Geometry: final body of the model. Coordinates: model frame, mm. A direction names the side the tool comes from. Give positions to 0.01 mm unless a question says otherwise; leave off trailing zeros. Write each loop counter-clockwise with the first axis right and the second up, starting at its lowest first coordinate (ties: lowest second). Pieces come first, ordered by that corner, then holes. Notation, with made-up numbers: M 79.25,76 L 124.25,76 A32 cw 124.25,105 Z; hole C -12.5,54 d4. An arc over 180 degrees is marked long. One line per question, with ' | ' between items.
from build123d import *

# Parameters (mm, degrees)
SKIZZE1_W                            = 238.8
SKIZZE1_H                            = 154.7
AUFSATZ_LINEAR_AUSTRAGEN1_DEPTH      = 3
SKIZZE2_W                            = 238.8
SKIZZE2_H                            = 154.7
SKIZZE2_W_2                          = 204.8
SKIZZE2_H_2                          = 120.7
SCHNITT_LINEAR_AUSTRAGEN2_DEPTH      = 2
VERRUNDUNG3_R                        = 8
F_3_0_3_DURCHMESSER_BOHRUNG1_D       = 3
SKIZZE6_W                            = 52
SKIZZE6_H                            = 44.7
SCHNITT_LINEAR_AUSTRAGEN3_DEPTH      = 285.546182543
SKIZZE7_W                            = 131.8
SKIZZE7_H                            = 87.7
SCHNITT_LINEAR_AUSTRAGEN4_DEPTH      = 285.546182543
SKIZZE5_W                            = 137.8
SKIZZE5_H                            = 93.7
SKIZZE5_W_2                          = 131.8
SKIZZE5_H_2                          = 87.7
AUFSATZ_LINEAR_AUSTRAGEN2_DEPTH      = 25
SCHNITT_LINEAR_AUSTRAGEN5_REACH      = 246.152
SKIZZE8_W                            = 40.7
SKIZZE8_H                            = 2
SKIZZE9_W                            = 43
SKIZZE9_H                            = 23
AUFSATZ_LINEAR_AUSTRAGEN3_DEPTH      = 4
F_3_4_3_4_DURCHMESSER_BOHRUNG1_D     = 3.4
F_3_4_3_4_DURCHMESSER_BOHRUNG1_DEPTH = 6
F_3_4_3_4_DURCHMESSER_BOHRUNG1_TIP   = 1.021463052
SCHNITT_LINEAR_AUSTRAGEN6_REACH      = 274.244
SKIZZE12_W                           = 43
SKIZZE12_H                           = 15.5
SKIZZE13_W                           = 5
SKIZZE13_H                           = 5
AUFSATZ_LINEAR_AUSTRAGEN4_DEPTH      = 15
F_3_4_3_4_DURCHMESSER_BOHRUNG2_D     = 3.4
F_3_4_3_4_DURCHMESSER_BOHRUNG2_DEPTH = 8
F_3_4_3_4_DURCHMESSER_BOHRUNG2_TIP   = 1.021463052
FASE1_SIZE                           = 5
VERRUNDUNG4_R                        = 3


with BuildPart() as part:
    # Skizze1 → Aufsatz-Linear austragen1 (new body)
    with BuildSketch(Plane(origin=(0, 0, 0), x_dir=(1, 0, 0), z_dir=(0, 1, 0))):
        with Locations((119.4, 77.35)):
            Rectangle(SKIZZE1_W, SKIZZE1_H)
    extrude(amount=AUFSATZ_LINEAR_AUSTRAGEN1_DEPTH)

    # Skizze2 → Schnitt-Linear austragen2 (cut)
    with BuildSketch(Plane(origin=(0, 3, 0), x_dir=(1, 0, 0), z_dir=(0, 1, 0))):
        with Locations((119.4, 77.35)):
            Rectangle(SKIZZE2_W, SKIZZE2_H)
        with Locations((119.4, 77.35)):
            Rectangle(SKIZZE2_W_2, SKIZZE2_H_2, mode=Mode.SUBTRACT)
    extrude(amount=-SCHNITT_LINEAR_AUSTRAGEN2_DEPTH, mode=Mode.SUBTRACT)

    # Verrundung3
    verrundung3_edges = [part.edges().sort_by_distance(p)[0] for p in [
        (0, 0.5, -154.7),
        (238.8, 0.5, -154.7),
        (238.8, 0.5, 0),
        (0, 0.5, 0),
    ]]
    fillet(verrundung3_edges, radius=VERRUNDUNG3_R)

    # Ø3.0 (3) Durchmesser Bohrung1 (through all)
    with Locations(Plane(origin=(0, 1, 0), x_dir=(1, 0, 0), z_dir=(0, 1, 0))):
        with Locations((13, 13), (135.8, 13), (225.8, 13), (225.8, 141.7), (135.8, 141.7), (13, 141.7)):
            Hole(F_3_0_3_DURCHMESSER_BOHRUNG1_D / 2)

    # Skizze6 → Schnitt-Linear austragen3 (cut, through all)
    with BuildSketch(Plane(origin=(0, 3, 0), x_dir=(1, 0, 0), z_dir=(0, 1, 0))):
        with Locations((26, 86.35)):
            Rectangle(SKIZZE6_W, SKIZZE6_H)
    extrude(amount=-SCHNITT_LINEAR_AUSTRAGEN3_DEPTH, mode=Mode.SUBTRACT)

    # Skizze7 → Schnitt-Linear austragen4 (cut, through all)
    with BuildSketch(Plane(origin=(0, 3, 0), x_dir=(1, 0, 0), z_dir=(0, 1, 0))):
        with Locations((120.9, 80.85)):
            Rectangle(SKIZZE7_W, SKIZZE7_H)
    extrude(amount=-SCHNITT_LINEAR_AUSTRAGEN4_DEPTH, mode=Mode.SUBTRACT)

    # Skizze5 → Aufsatz-Linear austragen2 (add)
    with BuildSketch(Plane(origin=(0, 3, 0), x_dir=(1, 0, 0), z_dir=(0, 1, 0))):
        with Locations((120.9, 80.85)):
            Rectangle(SKIZZE5_W, SKIZZE5_H)
        with Locations((120.9, 80.85)):
            Rectangle(SKIZZE5_W_2, SKIZZE5_H_2, mode=Mode.SUBTRACT)
    extrude(amount=AUFSATZ_LINEAR_AUSTRAGEN2_DEPTH)

    # Skizze8 → Schnitt-Linear austragen5 (cut, up to next)
    with BuildSketch(Plane.ZY.offset(-52), mode=Mode.PRIVATE) as schnitt_linear_austragen5_sk1:
        with Locations((-86.35, 1)):
            Rectangle(SKIZZE8_W, SKIZZE8_H)
    schnitt_linear_austragen5_tool1 = extrude(schnitt_linear_austragen5_sk1.sketch, amount=-SCHNITT_LINEAR_AUSTRAGEN5_REACH, mode=Mode.PRIVATE) & part.part
    add(schnitt_linear_austragen5_tool1.solids().sort_by_distance((52, 1, -86.35))[0], mode=Mode.SUBTRACT)

    # Skizze9 → Aufsatz-Linear austragen3 (add)
    with BuildSketch(Plane(origin=(0, 3, 0), x_dir=(1, 0, 0), z_dir=(0, 1, 0))):
        with Locations((119.4, 126.2)):
            Rectangle(SKIZZE9_W, SKIZZE9_H)
    extrude(amount=AUFSATZ_LINEAR_AUSTRAGEN3_DEPTH)

    # Ø3.4 (3.4) Durchmesser Bohrung1
    with Locations(Plane(origin=(0, 7, 0), x_dir=(1, 0, 0), z_dir=(0, 1, 0))):
        with Locations((101.9, 134.7), (136.9, 134.7), (136.9, 120.7), (101.9, 120.7)):
            Hole(F_3_4_3_4_DURCHMESSER_BOHRUNG1_D / 2, depth=F_3_4_3_4_DURCHMESSER_BOHRUNG1_DEPTH)
            with Locations((0, 0, -(F_3_4_3_4_DURCHMESSER_BOHRUNG1_DEPTH + F_3_4_3_4_DURCHMESSER_BOHRUNG1_TIP / 2))):  # 118° drill point
                Cone(0, F_3_4_3_4_DURCHMESSER_BOHRUNG1_D / 2, F_3_4_3_4_DURCHMESSER_BOHRUNG1_TIP, mode=Mode.SUBTRACT)

    # Skizze12 → Schnitt-Linear austragen6 (cut, up to next)
    with BuildSketch(Plane(origin=(0, 0, -127.7), x_dir=(-1, 0, 0), z_dir=(0, 0, -1)), mode=Mode.PRIVATE) as schnitt_linear_austragen6_sk1:
        with Locations((-119.4, 14.75)):
            Rectangle(SKIZZE12_W, SKIZZE12_H)
    schnitt_linear_austragen6_tool1 = extrude(schnitt_linear_austragen6_sk1.sketch, amount=-SCHNITT_LINEAR_AUSTRAGEN6_REACH, mode=Mode.PRIVATE) & part.part
    add(schnitt_linear_austragen6_tool1.solids().sort_by_distance((119.4, 14.75, -127.7))[0], mode=Mode.SUBTRACT)

    # Skizze13 → Aufsatz-Linear austragen4 (add)
    with BuildSketch(Plane(origin=(0, 28, 0), x_dir=(1, 0, 0), z_dir=(0, 1, 0))):
        with Locations((57.5, 122.2)):
            Rectangle(SKIZZE13_W, SKIZZE13_H)
        with Locations((184.3, 122.2)):
            Rectangle(SKIZZE13_W, SKIZZE13_H)
        with Locations((184.3, 39.5)):
            Rectangle(SKIZZE13_W, SKIZZE13_H)
        with Locations((57.5, 39.5)):
            Rectangle(SKIZZE13_W, SKIZZE13_H)
    extrude(amount=-AUFSATZ_LINEAR_AUSTRAGEN4_DEPTH)

    # Ø3.4 (3.4) Durchmesser Bohrung2
    with Locations(Plane(origin=(0, 28, 0), x_dir=(1, 0, 0), z_dir=(0, 1, 0))):
        with Locations((56, 123.7), (185.8, 123.7), (185.8, 38), (56, 38)):
            Hole(F_3_4_3_4_DURCHMESSER_BOHRUNG2_D / 2, depth=F_3_4_3_4_DURCHMESSER_BOHRUNG2_DEPTH)
            with Locations((0, 0, -(F_3_4_3_4_DURCHMESSER_BOHRUNG2_DEPTH + F_3_4_3_4_DURCHMESSER_BOHRUNG2_TIP / 2))):  # 118° drill point
                Cone(0, F_3_4_3_4_DURCHMESSER_BOHRUNG2_D / 2, F_3_4_3_4_DURCHMESSER_BOHRUNG2_TIP, mode=Mode.SUBTRACT)

    # Fase1
    fase1_edges = [part.edges().sort_by_distance(p)[0] for p in [
        (60, 13, -39.5),
        (181.8, 13, -39.5),
        (181.8, 13, -122.2),
        (60, 13, -122.2),
    ]]
    chamfer(fase1_edges, length=FASE1_SIZE - 0.0001)  # a hair under: the kernel refuses the full size

    # Verrundung4
    verrundung4_edges = [part.edges().sort_by_distance(p)[0] for p in [
        (52, 15.5, -127.7),
        (52, 15.5, -34),
        (189.8, 15.5, -34),
        (189.8, 15.5, -127.7),
    ]]
    fillet(verrundung4_edges, radius=VERRUNDUNG4_R)


solid = part.part
(1) Draft query along X for faces 4 (the face through (60, 23, -39)), 5 (the face through (2.281, 0.507, -2.406)), 6 (the face through (121, 28, -36)). Return one class per face: released by +X, released by -X, zero draft, split by the parting line, or undercut.
Working result:
face 4: undercut | face 5: released by -X | face 6: zero draft
(2) First-contact query: P1, Ø8.5, axis at y = 8, z = -81.5, coming from the +X side; P2, Ø5.5, axis at x = 57, y = 23, coming from the -Z side; P3, Ø1.5, axis at y = 3.5, z = -85, coming from the +X side; P4, Ø1.5, axis at x = 63, z = -39.5, coming from the -Y side. Flat tips, straight axial feed; report the tip coordinate or a pass-through.
Working result:
P1: stops at x = 189.8 | P2: stops at z = -127.7 | P3: stops at x = 221.8 | P4: passes through
(3) Set-up query: faces 1 (the face through (189.8, 15, -80)), 2 (the face through (119, 3, -120)), 3 (the face through (57, 22, -42)). Return all of +Z, -Z, +X, -X, +Y, -Y with unobstructed straight access to the full face (end or side cutting, diameter ignored); none if empty.
Working result:
face 1: +Z, -Z, +X, +Y | face 2: -Y | face 3: +Y, -Y
(4) Cut plane D-D, the plane x = 217.5. Return loops of the section in (y, z).
Working result:
outline: M 0,-154.7 L 1,-154.7 L 1,-137.7 L 3,-137.7 L 3,-17 L 1,-17 L 1,0 L 0,0 Z
(5) Cut plane C-C, the plane y = 9.5. Return loops of the section in (x, z).
Working result:
outline: M 52,-124.7 A3 ccw 55,-127.7 L 97.9,-127.7 L 97.9,-124.7 L 55,-124.7 L 55,-37 L 186.8,-37 L 186.8,-124.7 L 140.9,-124.7 L 140.9,-127.7 L 186.8,-127.7 A3 ccw 189.8,-124.7 L 189.8,-37 A3 ccw 186.8,-34 L 55,-34 A3 ccw 52,-37 Z
(6) Cut plane A-A, the plane z = -58.5. Return loops of the section in (x, y).
Working result:
outline: M 0,0 L 55,0 L 55,28 L 52,28 L 52,3 L 17,3 L 17,1 L 0,1 Z; M 186.8,0 L 238.8,0 L 238.8,1 L 221.8,1 L 221.8,3 L 189.8,3 L 189.8,28 L 186.8,28 Z
(7) Cut plane B-B, the plane x = 64. Return loops of the section in (y, z).
Working result:
outline: M 0,-154.7 L 1,-154.7 L 1,-137.7 L 3,-137.7 L 3,-127.7 L 28,-127.7 L 28,-124.7 L 0,-124.7 Z; M 0,-37 L 28,-37 L 28,-34 L 3,-34 L 3,-17 L 1,-17 L 1,0 L 0,0 Z
(8) Material intervals for L1, parallel to Z at x = 136.9, y = 3.6; L2, parallel to X at y = 24.5, z = -38; L3, parallel to X at y = 3.9, z = -134.7, sorted ascending. Write a range as [from, to].
Working result:
L1: z = [-137.7, -136.4], [-133, -122.4], [-119, -114.7], [-37, -34] | L2: x = [52, 54.3], [57.7, 60], [181.8, 184.1], [187.5, 189.8] | L3: x = [97.9, 100.2], [103.6, 135.2], [138.6, 140.9]
